Input: part model. Units: mm. Frame: model coordinates. Face numbers are marked on the shaded views. Give positions to 0.01 mm unless a question says otherwise; leave off trailing zeros. Write each loop counter-clockwise with the first axis right and the second up, starting at its lowest first coordinate (ties: lowest second). Pieces come first, ordered by that corner, then holes. Notation, with made-up numbers: M -14.75,29.5 L -4.75,29.5 A9 ccw -4.75,35.5 Z; hole C 43.25,-5 d1. An arc over 180 degrees is marked long. Use CSV: the item, a comma, the result in double quotes. Start each with the question number.
from build123d import *

# Parameters (mm, degrees)
SKETCH1_W               = 295
SKETCH1_H               = 292.1
BOSS_EXTRUDE1_DEPTH     = 88.69
BOSS_EXTRUDE1_DRAFT     = -2
SKETCH3_W               = 253.5
SKETCH3_H               = 252.5
CUT_EXTRUDE3_DEPTH      = 6.5
CUT_EXTRUDE3_DRAFT      = -2
SKETCH5_W               = 247
SKETCH5_H               = 247
CUT_EXTRUDE4_DEPTH      = 70.5
CUT_EXTRUDE4_DRAFT      = -2
CUT_EXTRUDE5_DEPTH      = 228.203831614
CUT_EXTRUDE5_DEPTH_BACK = 228.203831614
FILLET2_R               = 17.27
BOSS_EXTRUDE2_DEPTH     = 20.53
CUT_EXTRUDE6_REACH      = 337.359
SKETCH8_R               = 7
CUT_EXTRUDE7_DEPTH      = 5
CUT_EXTRUDE8_REACH      = 333.091
SKETCH9_R               = 1.75


with BuildPart() as part:
    # Sketch1 → Boss-Extrude1 (with draft: the straight prism first)
    with BuildSketch(Plane(origin=(0, 0, 0), x_dir=(1, 0, 0), z_dir=(0, 1, 0))):
        with Locations((2.25, 0)):
            Rectangle(SKETCH1_W, SKETCH1_H)
    extrude(amount=-BOSS_EXTRUDE1_DEPTH)
    # Boss-Extrude1: the draft: its side faces are tilted about the plane it starts from
    boss_extrude1_sides = [part.faces().sort_by_distance(p)[0] for p in [
        (2.25, -44.345, 146.05),
        (149.75, -44.345, 0),
        (2.25, -44.345, -146.05),
        (-145.25, -44.345, 0),
    ]]
    draft(boss_extrude1_sides, Plane(origin=(0, 0, 0), x_dir=(1, 0, 0), z_dir=(0, 1, 0)), BOSS_EXTRUDE1_DRAFT)


with BuildPart() as cut_extrude3_tool:
    # Sketch3 → Cut-Extrude3 (with draft: the straight prism first)
    with BuildSketch(Plane(origin=(0, 0, 0), x_dir=(1, 0, 0), z_dir=(0, 1, 0))):
        Rectangle(SKETCH3_W, SKETCH3_H)
    extrude(amount=-CUT_EXTRUDE3_DEPTH)
    # Cut-Extrude3: the draft: its side faces are tilted about the plane it starts from
    cut_extrude3_sides = [cut_extrude3_tool.faces().sort_by_distance(p)[0] for p in [
        (0, -3.25, 126.25),
        (126.75, -3.25, 0),
        (0, -3.25, -126.25),
        (-126.75, -3.25, 0),
    ]]
    draft(cut_extrude3_sides, Plane(origin=(0, 0, 0), x_dir=(1, 0, 0), z_dir=(0, 1, 0)), CUT_EXTRUDE3_DRAFT)


with BuildPart() as part_1:
    add(part.part)

    # Cut-Extrude3: cut by cut_extrude3_tool
    add(cut_extrude3_tool.part, mode=Mode.SUBTRACT)


with BuildPart() as cut_extrude4_tool:
    # Sketch5 → Cut-Extrude4 (with draft: the straight prism first)
    with BuildSketch(Plane(origin=(0, -6.5, 0), x_dir=(1, 0, 0), z_dir=(0, 1, 0))):
        Rectangle(SKETCH5_W, SKETCH5_H)
    extrude(amount=-CUT_EXTRUDE4_DEPTH)
    # Cut-Extrude4: the draft: its side faces are tilted about the plane it starts from
    cut_extrude4_sides = [cut_extrude4_tool.faces().sort_by_distance(p)[0] for p in [
        (0, -41.75, 123.5),
        (123.5, -41.75, 0),
        (0, -41.75, -123.5),
        (-123.5, -41.75, 0),
    ]]
    draft(cut_extrude4_sides, Plane(origin=(0, -6.5, 0), x_dir=(1, 0, 0), z_dir=(0, 1, 0)), CUT_EXTRUDE4_DRAFT)


with BuildPart() as part_2:
    add(part_1.part)

    # Cut-Extrude4: cut by cut_extrude4_tool
    add(cut_extrude4_tool.part, mode=Mode.SUBTRACT)

    # Sketch6 → Cut-Extrude5 (cut, two sides: drawn at the far end of the back side and taken through both)
    with BuildSketch(Plane.XY.offset(-CUT_EXTRUDE5_DEPTH_BACK)):
        Polygon((149.75, 0), (145, 0), (145, -88.69), (146.652876954, -88.69), align=None)
    extrude(amount=CUT_EXTRUDE5_DEPTH + CUT_EXTRUDE5_DEPTH_BACK, mode=Mode.SUBTRACT)

    # Fillet2
    fillet2_edges = [part_2.edges().sort_by_distance(p)[0] for p in [
        (-142.152876954, -88.69, 0),
        (1.423561523, -88.69, 142.952876954),
        (1.423561523, -88.69, -142.952876954),
        (-143.701438477, -44.345, 144.501438477),
        (-143.701438477, -44.345, -144.501438477),
    ]]
    fillet(fillet2_edges, radius=FILLET2_R)

    # Sketch7 → Boss-Extrude2 (add)
    with BuildSketch(Plane(origin=(0, 0, 0), x_dir=(1, 0, 0), z_dir=(0, 1, 0))):
        with BuildLine():
            Line((145, 128.78), (145, 146.05))
            Line((145, 146.05), (127.73, 146.05))
            ThreePointArc((127.73, 146.05), (139.941734111, 140.991734111), (145, 128.78))
        make_face()
        with BuildLine():
            Line((145, -146.05), (127.73, -146.05))
            ThreePointArc((127.73, -146.05), (139.941734111, -140.991734111), (145, -128.78))
            Line((145, -128.78), (145, -146.05))
        make_face()
    extrude(amount=BOSS_EXTRUDE2_DEPTH)

    # Sketch8 → Cut-Extrude6 (cut, up to next)
    with BuildSketch(Plane(origin=(-145.07308915, -5.066063906, 0), x_dir=(0, 0, 1), z_dir=(-0.9993908270190958, -0.03489949670250105, 0)), mode=Mode.PRIVATE) as cut_extrude6_sk1:
        with Locations(Location((-106.3, -19.400848104, 0), (0, 0, 270))):
            Circle(SKETCH8_R)
    cut_extrude6_tool1 = extrude(cut_extrude6_sk1.sketch, amount=-CUT_EXTRUDE6_REACH, mode=Mode.PRIVATE) & part_2.part
    add(cut_extrude6_tool1.solids().sort_by_distance((-144.396009, -24.455094, -106.3))[0], mode=Mode.SUBTRACT)

    # Sketch8_3 → Cut-Extrude7 (cut)
    with BuildSketch(Plane(origin=(-145.07308915, -5.066063906, 0), x_dir=(0, 0, 1), z_dir=(-0.9993908270190958, -0.03489949670250105, 0))):
        with BuildLine():
            ThreePointArc((-77, -17.550848104), (-76.707106781, -16.843741323), (-76, -16.550848104))
            Line((-76, -16.550848104), (-66.6, -16.550848104))
            ThreePointArc((-66.6, -16.550848104), (-65.892893219, -16.843741323), (-65.6, -17.550848104))
            Line((-65.6, -17.550848104), (-65.6, -21.250848104))
            ThreePointArc((-65.6, -21.250848104), (-65.892893219, -21.957954885), (-66.6, -22.250848104))
            Line((-66.6, -22.250848104), (-76, -22.250848104))
            ThreePointArc((-76, -22.250848104), (-76.707106781, -21.957954885), (-77, -21.250848104))
            Line((-77, -21.250848104), (-77, -17.550848104))
        make_face()
    extrude(amount=-CUT_EXTRUDE7_DEPTH, mode=Mode.SUBTRACT)

    # Sketch9 → Cut-Extrude8 (cut, up to next)
    with BuildSketch(Plane(origin=(-140.076135015, -4.891566422, 0), x_dir=(0, 0, 1), z_dir=(-0.9993908270190958, -0.03489949670250113, 0)), mode=Mode.PRIVATE) as cut_extrude8_sk1:
        with Locations(Location((-71.3, -19.400848104, 0), (0, 0, 270))):
            Circle(SKETCH9_R)
    cut_extrude8_tool1 = extrude(cut_extrude8_sk1.sketch, amount=-CUT_EXTRUDE8_REACH, mode=Mode.PRIVATE) & part_2.part
    add(cut_extrude8_tool1.solids().sort_by_distance((-139.399055, -24.280596, -71.3))[0], mode=Mode.SUBTRACT)


solid = part_2.part
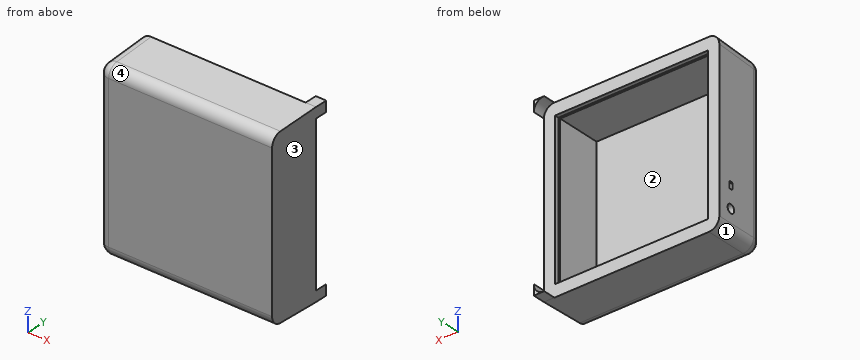
Q1. Section B-B, the plane x = 103.5. Return the cut outline in (y, z), and give its area (3 significant figures).
Q2. Section A-A, the plane z = -39. Return the cut outline in (x, y), and give its area (3 significant figures).
Q3. Material intervals for L1, parallel to Y at x = 41.5, z = 96; L2, parallel to Y at x = -65, z = 127.5; L3, parallel to X at y = -39, z = -59, sorted ascending. Write a range as [from, to].
Q4. First-contact query: pin 1 Ø8 at (y, z) = (-53, 46.5) entering from -X; pin 2 Ø12 at (x, y) = (35, -35.5) entering from +Z; pin 3 Ø1.9 at (x, y) = (-143, -24) entering from +Z. Flat tips, straight axial feed; report the tip coordinate or a pass-through.
Q5. Pull-direction query (Z, two-part tool) for the marked faces 1, 2, 3 and 4; classes: released by +Z, released by -Z, zero draft, split by the parting line, or undercut.
Check result:
1,outline,"M -88.69,-126.28 A17.27 ccw -72.02,-143.53 L 0,-146.05 L 0,-126.25 L -6.5,-126.02 L -6.5,-123.5 L -77,-121.04 L -77,121.04 L -6.5,123.5 L -6.5,126.02 L 0,126.25 L 0,146.05 L -72.02,143.53 A17.27 ccw -88.69,126.28 Z"
1,area,"6,630 mm²"
2,outline,"M -145.25,0 L -142.73,-72.02 A17.27 ccw -125.48,-88.69 L 145,-88.69 L 145,0 L 126.75,0 L 126.52,-6.5 L 123.5,-6.5 L 121.04,-77 L -121.04,-77 L -123.5,-6.5 L -126.52,-6.5 L -126.75,0 Z"
2,area,"6,660 mm²"
3,L1,"y = [-88.69, -77]"
3,L2,"y = [-88.65, 0]"
3,L3,"x = [-143.89, -122.37], [122.37, 145]"
4,pin 1,"stops at x = -143.54"
4,pin 2,"stops at z = 145.02"
4,pin 3,"stops at z = 136.67"
5,face 1,"released by -Z"
5,face 2,"undercut"
5,face 3,"zero draft"
5,face 4,"released by +Z"
